```python
from build123d import *

# Parameters (mm, degrees)
F0_R          = 3.175
F1_DEPTH      = 12.7
F2_R          = 4.7625
F2_R_2        = 3.175
F3_DEPTH      = 12.7
F4_R          = 0.254
F5_DEPTH      = 25.4
F6_R          = 3.7465
F6_R_2        = 0.254
F7_DEPTH      = 6.35
F8_R          = 0.79375
F9_DEPTH      = 4.7635
F9_DEPTH_BACK = 4.7635


with BuildPart() as f1:
    # F0 (on Top) → F1 (new body)
    with BuildSketch(Plane.XY):
        Circle(F0_R)
    extrude(amount=F1_DEPTH)

    # F2 (on face) → F3 (join)
    with BuildSketch(Plane(origin=(0, 0, 0), x_dir=(1, 0, 0), z_dir=(0, 0, -1))):
        Circle(F2_R)
        Circle(F2_R_2, mode=Mode.SUBTRACT)
        Circle(F2_R_2)
    extrude(amount=F3_DEPTH)

    # F4 (on face) → F5 (cut)
    with BuildSketch(Plane(origin=(0, 0, -12.7), x_dir=(1, 0, 0), z_dir=(0, 0, -1))):
        Circle(F4_R)
    extrude(amount=-F5_DEPTH, mode=Mode.SUBTRACT)

    # F6 (on face) → F7 (cut)
    with BuildSketch(Plane(origin=(0, 0, -12.7), x_dir=(1, 0, 0), z_dir=(0, 0, -1))):
        Circle(F6_R)
        Circle(F6_R_2, mode=Mode.SUBTRACT)
    extrude(amount=-F7_DEPTH, mode=Mode.SUBTRACT)

    # F8 (on Right) → F9 (cut, two sides)
    with BuildSketch(Plane.YZ) as f9_sk:
        with Locations((0, -1.6002)):
            Circle(F8_R)
    extrude(amount=-F9_DEPTH, mode=Mode.SUBTRACT)
    extrude(f9_sk.sketch, amount=F9_DEPTH_BACK, mode=Mode.SUBTRACT)


solid = f1.part
```
The model under review builds one solid part; all positions refer to its coordinate system, in mm. A direction names the side the tool comes from. Give positions to 0.01 mm unless a question says otherwise; leave off trailing zeros. Write each loop counter-clockwise with the first axis right and the second up, starting at its lowest first coordinate (ties: lowest second). Pieces come first, ordered by that corner, then holes. Notation, with made-up numbers: M 53.25,-37.75 L 68.25,-37.75 A10 cw 68.25,-24.75 Z; hole C 66,81.5 d8. An arc over 180 degrees is marked long. Answer in a Markdown table with one row per item.
Item 1: Add section D-D on y = -3.5. Give the boundary of the cut face in (x, z), plus the area to 3 significant figures.
Check sheet entries:
| item | result |
|---|---|
| outline | M -3.23,-12.7 L -1.34,-12.7 L -1.34,-6.35 L 1.34,-6.35 L 1.34,-12.7 L 3.23,-12.7 L 3.23,0 L -3.23,0 Z |
| area | 65.1 mm2 |
Item 2: Add section A-A on y = 0. State how many separate pieces and enclosed holes the cut face has, plus the area to 3 significant figures.
Check sheet entries:
| item | result |
|---|---|
| separate pieces | 4 |
| enclosed holes | 0 |
| area | 130 mm2 |
Item 3: Add section C-C on z = -4.25. Give the boundary of the cut face in (x, y) (1 decimal), plus the area to 3 significant figures.
Check sheet entries:
| item | result |
|---|---|
| outline | C 0,0 d9.5; hole C 0,0 d0.5 |
| area | 71.1 mm2 |
Item 4: Tool access review of faces 4 (the face through (-4, 1, -12.7)), 5 (the face through (-0.69, -3.1, 6.26)), 6 (the face through (-0.488, -3.715, -9.569)): name each direction out of +Z, -Z, +X, -X, +Y, -Y from which nothing blocks a thin tool from reaching the whole face with its end or side.
Check sheet entries:
| item | result |
|---|---|
| face 4 | -Z, +X, -X, +Y, -Y |
| face 5 | +Z |
| face 6 | -Z |
Item 5: Add section B-B on x = -1.5. Give the boundary of the cut face in (y, z).
Check sheet entries:
| item | result |
|---|---|
| outline | M -4.52,-12.7 L -3.43,-12.7 L -3.43,-6.35 L 3.43,-6.35 L 3.43,-12.7 L 4.52,-12.7 L 4.52,0 L 2.8,0 L 2.8,12.7 L -2.8,12.7 L -2.8,0 L -4.52,0 Z; hole C 0,-1.6 d1.59 |
Item 6: For line 1 along Y through (x, z) = (0, -9.5); line 2 along Z through (x, y) = (-2.7, 0); line 3 along Y through (x, z) = (0, 5) (3 decimals), list the stretches that pass through material, from the lowest coordinate up.
Check sheet entries:
| item | result |
|---|---|
| line 1 | -4.76 to -3.75, 3.75 to 4.76 |
| line 2 | -6.35 to -2.39, -0.81 to 12.7 |
| line 3 | -3.175 to -0.254, 0.254 to 3.175 |
Item 7: Draft analysis for pull direction X (two halves, no side actions). For faces 1 (the face through (4.543, -1.431, -6.261)), 2 (the face through (0, 1, -6.35)), 3 (the face through (1, 0, 12.7)), state which applies: +X half, -X half, draft (parallel to the pull), parting line (faces both ways), or undercut.
Check sheet entries:
| item | result |
|---|---|
| face 1 | parting line |
| face 2 | undercut |
| face 3 | draft |
Item 8: For P1, Ø1, axis at x = 2.5, z = -8, coming from the +Y side; P2, Ø3, axis at y = 0.5, z = -10, coming from the +X side; P3, Ø3.5, axis at x = -1.5, y = -0.5, coming from the -Z side; P4, Ø1.5, axis at x = 0.5, z = 7.5, coming from the -Y side (3 decimals), all flat-tipped, find the tip position at first contact; note any pin that passes through.
Check sheet entries:
| item | result |
|---|---|
| P1 | y = 4.32 |
| P2 | x = 4.76 |
| P3 | z = -6.35 |
| P4 | y = -3.175 |
